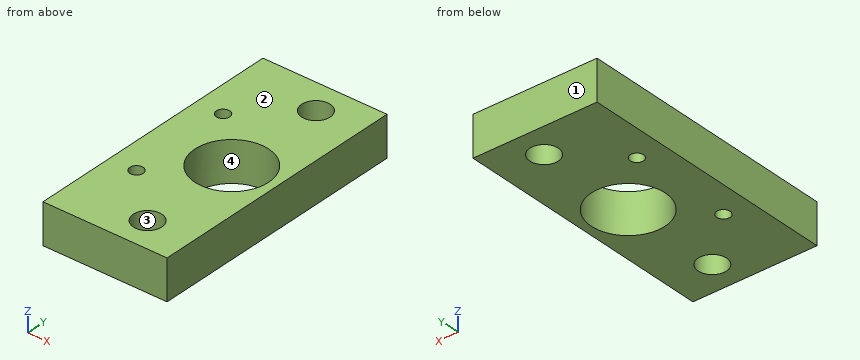
from build123d import *

# Parameters (mm, degrees)
F0_R     = 2
F0_R_2   = 4.25
F0_R_3   = 11
F1_DEPTH = 12


with BuildPart() as f1:
    # F0 (on Top) → F1 (new body)
    with BuildSketch(Plane.XY):
        Polygon((13.5, -39.4), (13.5, -15.5), (13.5, 15.5), (13.5, 39.4), (-23.5, 39.4), (-23.5, 19.5), (-23.5, -19.5), (-23.5, -39.4), align=None)
        with Locations((-15.5, -15.5)):
            Circle(F0_R, mode=Mode.SUBTRACT)
        with Locations((0, -30.15)):
            Circle(F0_R_2, mode=Mode.SUBTRACT)
        with Locations((-15.5, 15.5)):
            Circle(F0_R, mode=Mode.SUBTRACT)
        Circle(F0_R_3, mode=Mode.SUBTRACT)
        with Locations((0, 30.15)):
            Circle(F0_R_2, mode=Mode.SUBTRACT)
    extrude(amount=F1_DEPTH)


solid = f1.part
For this review, take the finished solid that the model builds, in its own axes (mm). Face numbers are marked on the shaded views. Round coordinates to 2 decimals unless told otherwise and drop trailing zeros. Loops run counter-clockwise (first coordinate to the right, second up) from the corner with the lowest first, then second, coordinate; pieces in that order, holes last. Notation, with made-up numbers: (54, 84.5) - (91, 84.5) arc R18 ccw to (91, 96.5) - close; hole circle Ø5 at (62, 52). An arc over 180 degrees is marked (long way). One line per question, with ' | ' between items.
Q1. The part is to be moulded in two halves that separate along Y. For the marked faces 1, 2, 3 and 4, say which applies: released by +Y, released by -Y, zero draft, split by the parting line, or undercut.
Taken from the geometry:
face 1: released by +Y | face 2: zero draft | face 3: undercut | face 4: undercut
Q2. Take a section at B-B (x = -15.5). Give the boundary of the cut face in (y, z).
Taken from the geometry:
outline: (-39.4, 0) - (-17.5, 0) - (-17.5, 12) - (-39.4, 12) - close; (-13.5, 0) - (13.5, 0) - (13.5, 12) - (-13.5, 12) - close; (17.5, 0) - (39.4, 0) - (39.4, 12) - (17.5, 12) - close
Q3. For pin 1 (5 mm diameter, centred on x = 0, y = 30.15, fed in from +Z), flat-tipped, find the tip position at first contact; note if it passes through.
Taken from the geometry:
pin 1: passes through
Q4. Take a section at C-C (z = 5.75). Give the boundary of the cut face in (x, y), and give its area (3 significant figures).
Taken from the geometry:
outline: (-23.5, -39.4) - (13.5, -39.4) - (13.5, 39.4) - (-23.5, 39.4) - close; hole circle Ø4 at (-15.5, -15.5); hole circle Ø4 at (-15.5, 15.5); hole circle Ø22 at (0, 0); hole circle Ø8.5 at (0, -30.15); hole circle Ø8.5 at (0, 30.15) | area: 2,400 mm²
Q5. Take a section at D-D (x = 7). Give the boundary of the cut face in (y, z).
Taken from the geometry:
outline: (-39.4, 0) - (-8.49, 0) - (-8.49, 12) - (-39.4, 12) - close; (8.49, 0) - (39.4, 0) - (39.4, 12) - (8.49, 12) - close
Q6. For line 1 along Y through (x, z) = (0, 10.75); line 2 along Y through (x, z) = (-15.5, 4); line 3 along Y through (x, z) = (-3.5, 10.5), list the stretches that pass through material, from the lowest coordinate up. Write a range as [from, to].
Taken from the geometry:
line 1: y = [-39.4, -34.4], [-25.9, -11], [11, 25.9], [34.4, 39.4] | line 2: y = [-39.4, -17.5], [-13.5, 13.5], [17.5, 39.4] | line 3: y = [-39.4, -32.56], [-27.74, -10.43], [10.43, 27.74], [32.56, 39.4]
Q7. Take a section at A-A (y = 30.15). Give the boundary of the cut face in (x, z).
Taken from the geometry:
outline: (-23.5, 0) - (-4.25, 0) - (-4.25, 12) - (-23.5, 12) - close; (4.25, 0) - (13.5, 0) - (13.5, 12) - (4.25, 12) - close
